Autodesk Inventor part; units mm, degrees
ref_plane "YZ Plane" through (0, 0, 0) normal (1, 0, 0) x (0, 1, 0)
ref_plane "XZ Plane" through (0, 0, 0) normal (0, 1, 0) x (-1, 0, 0)
ref_plane "XY Plane" through (0, 0, 0) normal (0, 0, 1) x (1, 0, 0)
sketch "Sketch1" plane through (0, 0, 0) normal (0, 1, 0) x (-1, 0, 0)
  line L0 (0, 0) -> (200, 0)
  line L1 (200, 0) -> (200, -30)
  line L2 (200, -30) -> (0, -30)
  line L3 (0, -30) -> (0, 0)
  line L4 (10, -15) -> (190, -15) construction
  line L5 (10, -13) -> (190, -13)
  line L6 (190, -17) -> (10, -17)
  arc A0 (10, -13) -> (10, -17) centre (10, -15) ccw
  arc A1 (190, -17) -> (190, -13) centre (190, -15) ccw
  point P0 (100, -15)
  dimension "d0" = 200
  dimension "d1" = 30
  dimension "d2" = 2
  dimension "d3" = 180
  dimension "d4" = 10
  dimension "d5" = 15
extrude "Extrusion1" add sketch "Sketch1" along normal blind 10
sketch "Sketch2" plane through (0, 0, 0) normal (0, -1, 0) x (1, 0, 0)
  arc A0 (-190, -13) -> (-190, -17) centre (-190, -15) ccw
  line L0 (-190, -15) -> (-10, -15) construction
  line L1 (-190, -17) -> (-10, -17)
  line L2 (-190, -21) -> (-10, -21)
  line L3 (-10, -9) -> (-190, -9)
  arc A1 (-190, -9) -> (-190, -21) centre (-190, -15) ccw
  arc A2 (-10, -21) -> (-10, -9) centre (-10, -15) ccw
  arc A3 (-10, -17) -> (-10, -13) centre (-10, -15) ccw
  point P0 (0, 0)
  point P1 (-100, -15)
  dimension "d10" = 12
extrude "Extrusion2" cut sketch "Sketch2" against normal blind 9
sketch "Sketch3" plane through (0, 10, 0) normal (0, 1, 0) x (1, 0, 0)
  line L0 (-200, 0) -> (0, 0)
  line L1 (0, 0) -> (0, 30)
  line L2 (0, 30) -> (-200, 30)
  line L3 (-200, 30) -> (-200, 0)
  line L4 (0, 30) -> (-200, 30)
  line L5 (-200, 30) -> (-200, 28)
  line L6 (-200, 28) -> (0, 28)
  line L7 (0, 28) -> (0, 30)
  point P0 (0, 28)
  dimension "d20" = 2
extrude "Extrusion3" add sketch "Sketch3" along normal blind 2 contours L3 L2 L1 L6
equation "\"d3\" = d0 - 2 * d4"
properties part number "SolderSupport" material "Aluminum"
CAD build for the part. Positions are in the model's coordinates, mm. A direction names the side the tool comes from. Round coordinates to 2 decimals unless told otherwise and drop trailing zeros. Order: outer loops, then holes, each group sorted by start corner. A loop starts at its lowest first (then second) coordinate and runs counter-clockwise, first axis right, second up.
Item 1: Tool access for faces 1 (the face through (0, 6, -15)), 2 (the face through (-196, 4, -15)), 3 (the face through (-99, 10, -11)): list every direction of +Z, -Z, +X, -X, +Y, -Y with a clear straight run to the whole face (end or side of a thin tool).
Item 2: Probe line 1 along Z through (x, y) = (-138.5, 3.75); line 2 along X through (y, z) = (3.75, -15); line 3 along Y through (x, z) = (-154, -6.25). List the from-to ranges inside material, lowest first.
Item 3: Saw through at B-B on z = -15. Write the cut outline in (x, y), then the cut area to 3 significant figures.
Item 4: Saw through at C-C on y = 3.5. Write the cut outline in (x, z).
Item 5: Mould opens along X. For faces 4 (the face through (-200, 6, -15)), 5 (the face through (-101, 9, -18)), 6 (the face through (-99, 0, -8)) say: pulls with the +X half, pulls with the -X half, needs draft (parallel to the pull), parting line crosses it, or undercut.
Item 6: Pin check, flat tips, straight feed: pin 1 (2 mm diameter, centred on x = -142.5, y = 11.5, fed in from +Z); pin 2 (1 mm diameter, centred on y = 3.5, z = -25.5, fed in from +X). Stop position of each tip, or through.
Item 7: Saw through at A-A on x = -166. Write the cut outline in (y, z), then the cut area to 3 significant figures.
Item 8: Saw through at D-D on z = -24. Write the cut outline in (x, y), then the cut area to 3 significant figures.
Reported:
1. face 1: +Z, -Z, +X, +Y, -Y
1. face 2: -Y
1. face 3: +Z, +X, -X, +Y
2. line 1: z = -30 to -21, -9 to 0
2. line 2: x = -200 to -196, -4 to 0
2. line 3: y = 0 to 10
3. outline: (-200, 0) - (-196, 0) - (-196, 9) - (-192, 9) - (-192, 10) - (-200, 10) - close; (-8, 9) - (-4, 9) - (-4, 0) - (0, 0) - (0, 10) - (-8, 10) - close
3. area: 88.0 mm2
4. outline: (-200, -30) - (0, -30) - (0, 0) - (-200, 0) - close; hole (-190, -21) - (-10, -21) arc R6 ccw to (-10, -9) - (-190, -9) arc R6 ccw to start
5. face 4: pulls with the -X half
5. face 5: undercut
5. face 6: needs draft
6. pin 1: stops at z = -28
6. pin 2: stops at x = 0
7. outline: (0, -30) - (12, -30) - (12, -28) - (10, -28) - (10, -17) - (9, -17) - (9, -21) - (0, -21) - close; (0, -9) - (9, -9) - (9, -13) - (10, -13) - (10, 0) - (0, 0) - close
7. area: 192 mm2
8. outline: (-200, 0) - (0, 0) - (0, 10) - (-200, 10) - close
8. area: 2,000 mm2
